Could you check a few things on this model? Use its own coordinates, in mm. A direction names the side the tool comes from. Give positions to 0.01 mm unless a question says otherwise; leave off trailing zeros. Loops run counter-clockwise (first coordinate to the right, second up) from the corner with the lowest first, then second, coordinate; pieces in that order, holes last. Notation, with made-up numbers: M -20.5,46 L 15.5,46 A13 cw 15.5,64 Z; hole C 16.25,34 d10. An arc over 180 degrees is marked long. Use a Markdown table: item, result. Add a question column.
1) Will these pins go through, and if not, where does the flat tip stop? pin 1 Ø9 at (y, z) = (3.5, 6) entering from -X; pin 2 Ø4 at (y, z) = (20.5, -8) entering from -X; pin 3 Ø8 at (y, z) = (-3, 6.5) entering from -X; pin 4 Ø13.5 at (x, y) = (-12, 3) entering from -Z.
2) Suppose I cut it at D-D on x = 8.5. List the corners of the cut face in (y, z) for me, and give its area (3 significant figures).
3) If I drill on line 1 along X through (y, z) = (-5.5, -12.5); line 2 along X through (y, z) = (-2, 3); line 3 along Y through (x, z) = (-15.5, 3.5), over which ranges is the centre line in solid material (lowest first)? Write a range as [from, to].
4) Which directions (+Z, -Z, +X, -X, +Y, -Y) give clear straight access to the entire face, cutting with the end or side of a thin tool? Please do faces 1 (the flat face through (-6.5, -7.1, 1.5)), 2 (the flat face through (-6.5, -7.1, 9.5)), 3 (the flat face through (1, -4, 0)).
5) Suppose I cut it at B-B on y = 11.5. List the corners of the cut face in (x, z) for me, and give its area (3 significant figures).
6) Suppose I cut it at A-A on z = 5.5. List the corners of the cut face in (x, y) for me.
7) Suppose I cut it at C-C on x = -5. List the corners of the cut face in (y, z) for me.
```python
from build123d import *

# Parameters (mm, degrees)
PAD_DEPTH    = 11
CHAMFER_SIZE = 3
FILLET_R     = 2
SKETCH001_W  = 39.802324
SKETCH001_H  = 56.00523
POCKET_DEPTH = 50
SKETCH002_W  = 40
SKETCH002_H  = 40
PAD001_DEPTH = 2
FILLET001_R  = 3


with BuildPart() as part:
    # Sketch → Pad (new body)
    with BuildSketch(Plane.XY):
        Polygon((-22.800474, -3.599016), (-22.800474, -8.599016), (10.199526, -8.599016), (10.199526, 18.400984), (28.199526, 18.400984), (28.199526, -8.599016), (31.199526, -8.599016), (31.199526, 21.400984), (7.199526, 21.400984), (7.199526, -3.599016), align=None)
    extrude(amount=PAD_DEPTH)

    # Chamfer
    chamfer_edges = [part.edges().sort_by_distance(p)[0] for p in [
        (-6.300474, -8.599016, 0),
        (-6.300474, -8.599016, 11),
    ]]
    chamfer(chamfer_edges, length=CHAMFER_SIZE)

    # Fillet
    fillet_edges = [part.edges().sort_by_distance(p)[0] for p in [
        (31.199526, 21.400984, 5.5),
        (7.199526, 21.400984, 5.5),
    ]]
    fillet(fillet_edges, radius=FILLET_R)

    # Sketch001 (on Face14 of Fillet) → Pocket (cut)
    with BuildSketch(Plane.XY.offset(11)):
        with Locations((30.100688, 5.3986)):
            Rectangle(SKETCH001_W, SKETCH001_H)
    extrude(amount=-POCKET_DEPTH, mode=Mode.SUBTRACT)

    # Sketch002 (on Face5 of Pocket) → Pad001 (join)
    with BuildSketch(Plane.YZ.offset(10.199526)):
        with Locations((11.400984, 5)):
            Rectangle(SKETCH002_W, SKETCH002_H)
    extrude(amount=PAD001_DEPTH)

    # Fillet001
    fillet001_edges = [part.edges().sort_by_distance(p)[0] for p in [
        (11.199526, 31.400984, 25),
        (11.199526, 31.400984, -15),
        (11.199526, -8.599016, -15),
        (11.199526, -8.599016, 25),
    ]]
    fillet(fillet001_edges, radius=FILLET001_R)


solid = part.part
```
Answer block:
| question | item | result |
|---|---|---|
| 1 | pin 1 | stops at x = 7.2 |
| 1 | pin 2 | stops at x = 10.2 |
| 1 | pin 3 | stops at x = -22.8 |
| 1 | pin 4 | stops at z = 0 |
| 2 | outline | M -8.6,3 L -5.6,0 L 21.27,0 L 21.27,11 L -5.6,11 L -8.6,8 Z |
| 2 | area | 320 mm^2 |
| 3 | line 1 | x = [10.2, 12.2] |
| 3 | line 2 | x = [7.2, 12.2] |
| 3 | line 3 | y = [-8.6, -3.6] |
| 4 | face 1 | -Z, -X, -Y |
| 4 | face 2 | +Z, -X, -Y |
| 4 | face 3 | -Z, -X, +Y, -Y |
| 5 | outline | M 7.2,0 L 10.2,0 L 10.2,-15 L 12.2,-15 L 12.2,25 L 10.2,25 L 10.2,11 L 7.2,11 Z |
| 5 | area | 113 mm^2 |
| 6 | outline | M -22.8,-8.6 L 12.2,-8.6 L 12.2,31.4 L 10.2,31.4 L 10.2,21.4 L 9.2,21.4 A2 ccw 7.2,19.4 L 7.2,-3.6 L -22.8,-3.6 Z |
| 7 | outline | M -8.6,3 L -5.6,0 L -3.6,0 L -3.6,11 L -5.6,11 L -8.6,8 Z |
